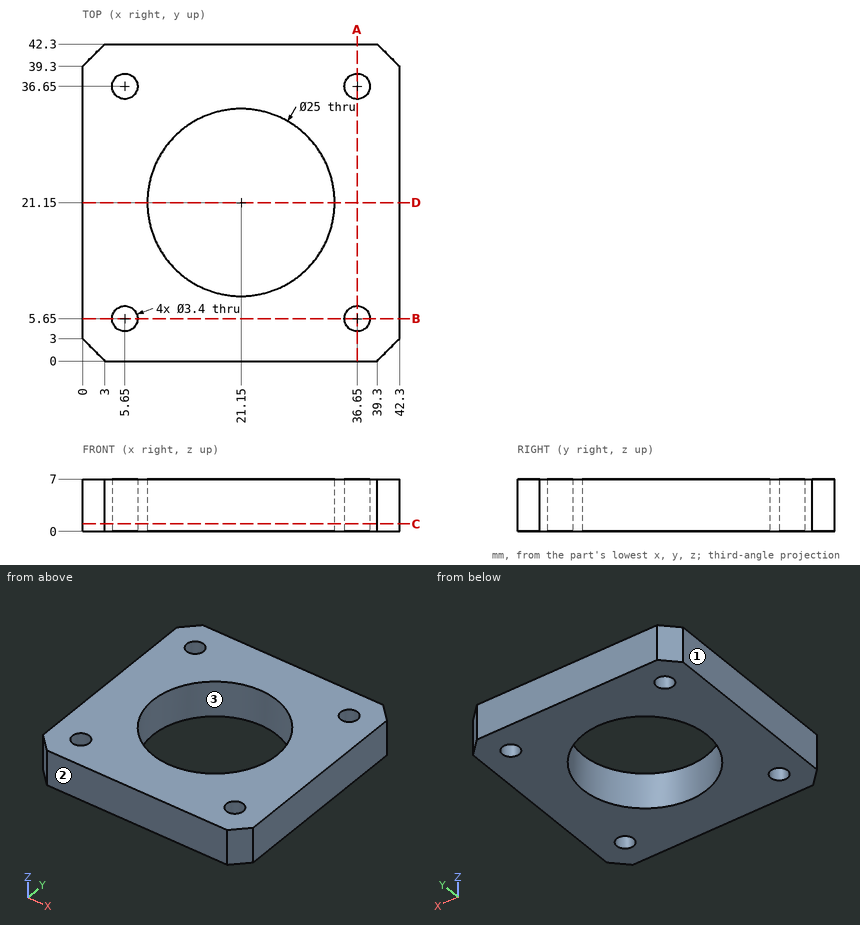
Source: three-view drawing plus pictorial views. Frame: mm from the lowest corner of the part. Give positions to 0.01 mm unless a question says otherwise; leave off trailing zeros. Order: outer loops, then holes, each group sorted by start corner. A loop starts at its lowest first (then second) coordinate and runs counter-clockwise, first axis right, second up. Notation, with made-up numbers: M 29.25,-20 L 71.25,-20 A37 ccw 71.25,17 Z; hole C -3.5,6.5 d3. An arc over 180 degrees is marked long. One line per question, with ' | ' between items. Start each with the question number.
1. Section query A-A (x = 36.65). Return the cut outline in (y, z), and give its area (4 significant figures).
2. Pull-direction query (Y, two-part tool) for the marked faces 1, 2 and 3; classes: released by +Y, released by -Y, zero draft, split by the parting line, or undercut.
3. First-contact query: pin 1 Ø2 at (x, y) = (5.65, 36.65) entering from -Z. Flat tip, straight axial feed; report the tip coordinate or a pass-through.
4. Material intervals for probe 1 along Y at (x, z) = (5.65, 5.25); probe 2 along Y at (x, z) = (5, 3.25), sorted ascending. Write a range as [from, to].
5. Section query C-C (z = 1). Return the cut outline in (x, y), and give its area (3 significant figures).
6. Section query D-D (y = 21.15). Return the cut outline in (x, z).
Here are the results:
1) outline: M 0,0 L 3.95,0 L 3.95,7 L 0,7 Z; M 7.35,0 L 34.95,0 L 34.95,7 L 7.35,7 Z; M 38.35,0 L 42.3,0 L 42.3,7 L 38.35,7 Z | area: 248.5 mm²
2) face 1: zero draft | face 2: released by -Y | face 3: undercut
3) pin 1: through
4) probe 1: [0, 3.95], [7.35, 34.95], [38.35, 42.3] | probe 2: [0, 4.08], [7.22, 35.08], [38.22, 42.3]
5) outline: M 0,3 L 3,0 L 39.3,0 L 42.3,3 L 42.3,39.3 L 39.3,42.3 L 3,42.3 L 0,39.3 Z; hole C 5.65,5.65 d3.4; hole C 5.65,36.65 d3.4; hole C 21.15,21.15 d25; hole C 36.65,5.65 d3.4; hole C 36.65,36.65 d3.4 | area: 1,240 mm²
6) outline: M 0,0 L 8.65,0 L 8.65,7 L 0,7 Z; M 33.65,0 L 42.3,0 L 42.3,7 L 33.65,7 Z
